For this review, take the finished solid that the model builds, in its own axes (mm). Coordinates: 2 decimals unless noted, no trailing zeros. Use one line per item in the form item = value. Start each with the question number.
1) Mouldability with a two-part tool opening along Z and no side actions: class faces 1 (the cylindrical face through (119.834, 1.479, 96.347)), 2 (the flat face through (119, 0, 49)) as pulls with the +Z half, pulls with the -Z half, needs draft (parallel to the pull), parting line crosses it, or undercut.
2) For L1, parallel to X at y = 0.6, z = 25; L2, parallel to X at y = 1.6, z = 5; L3, parallel to X at y = 1.9, z = 85, list the stretches that pass through material, from the lowest coordinate up. Write a range as from..to.
3) Insertion check: P1, Ø2.5, axis at x = 5, z = 5, coming from the +Y side. The pin has a flat end and moves straight along its axis. Give the tip position at first contact, or say it passes through.
```python
from build123d import *

# Parameters (mm, degrees)
SKETCH_181_W    = 243.2
SKETCH_181_H    = 100
SKETCH_181_R    = 1.8
SKETCH_181_R_2  = 2
EXTRUDE_3_DEPTH = 3


with BuildPart() as part:
    # Sketch 181 → 凸台-拉伸3 (new body)
    with BuildSketch(Plane(origin=(0, 0, 0), x_dir=(1, 0, 0), z_dir=(0, 1, 0))):
        with Locations((120.6, -50)):
            Rectangle(SKETCH_181_W, SKETCH_181_H)
        with Locations(Location((73.049576153, -12.361926171, 0), (0, 0, 270))):  # turned: the seam where the file's is
            Circle(SKETCH_181_R, mode=Mode.SUBTRACT)
        with Locations(Location((73.495550598, -83.360525501, 0), (0, 0, 270))):  # turned: the seam where the file's is
            Circle(SKETCH_181_R, mode=Mode.SUBTRACT)
        with Locations(Location((163.495550598, -12.360525501, 0), (0, 0, 270))):  # turned: the seam where the file's is
            Circle(SKETCH_181_R, mode=Mode.SUBTRACT)
        with Locations(Location((163.495550598, -83.360525501, 0), (0, 0, 270))):  # turned: the seam where the file's is
            Circle(SKETCH_181_R, mode=Mode.SUBTRACT)
        with Locations(Location((10.091186927, -32, 0), (0, 0, 270))):  # turned: the seam where the file's is
            Circle(SKETCH_181_R, mode=Mode.SUBTRACT)
        with Locations(Location((10.522883477, -64.497132767, 0), (0, 0, 270))):  # turned: the seam where the file's is
            Circle(SKETCH_181_R, mode=Mode.SUBTRACT)
        with Locations(Location((52.091186927, -32, 0), (0, 0, 270))):  # turned: the seam where the file's is
            Circle(SKETCH_181_R, mode=Mode.SUBTRACT)
        with Locations(Location((52.091186927, -64.497132767, 0), (0, 0, 270))):  # turned: the seam where the file's is
            Circle(SKETCH_181_R, mode=Mode.SUBTRACT)
        with Locations(Location((120.6, -5, 0), (0, 0, 270))):  # turned: the seam where the file's is
            Circle(SKETCH_181_R_2, mode=Mode.SUBTRACT)
        with Locations(Location((120.6, -94.5, 0), (0, 0, 270))):  # turned: the seam where the file's is
            Circle(SKETCH_181_R_2, mode=Mode.SUBTRACT)
        with Locations(Location((5, -5, 0), (0, 0, 270))):  # turned: the seam where the file's is
            Circle(SKETCH_181_R_2, mode=Mode.SUBTRACT)
        with Locations(Location((5, -94.5, 0), (0, 0, 270))):  # turned: the seam where the file's is
            Circle(SKETCH_181_R_2, mode=Mode.SUBTRACT)
        with Locations(Location((236.2, -5, 0), (0, 0, 270))):  # turned: the seam where the file's is
            Circle(SKETCH_181_R_2, mode=Mode.SUBTRACT)
        with Locations(Location((236.2, -94.5, 0), (0, 0, 270))):  # turned: the seam where the file's is
            Circle(SKETCH_181_R_2, mode=Mode.SUBTRACT)
        with Locations(Location((231.695550598, -25, 0), (0, 0, 270))):  # turned: the seam where the file's is
            Circle(SKETCH_181_R, mode=Mode.SUBTRACT)
        with Locations(Location((231.695550598, -74, 0), (0, 0, 270))):  # turned: the seam where the file's is
            Circle(SKETCH_181_R, mode=Mode.SUBTRACT)
        with Locations(Location((178.495550598, -74, 0), (0, 0, 270))):  # turned: the seam where the file's is
            Circle(SKETCH_181_R, mode=Mode.SUBTRACT)
        with Locations(Location((178.495550598, -25, 0), (0, 0, 270))):  # turned: the seam where the file's is
            Circle(SKETCH_181_R, mode=Mode.SUBTRACT)
    extrude(amount=EXTRUDE_3_DEPTH)


solid = part.part
```
Determined:
q1.face_1 = undercut
q1.face_2 = needs draft
q2.L1 = -1..176.7, 180.3..229.9, 233.5..242.2
q2.L2 = -1..3, 7..118.6, 122.6..234.2, 238.2..242.2
q2.L3 = -1..72.75, 74.24..162.75, 164.24..242.2
q3.P1 = through
